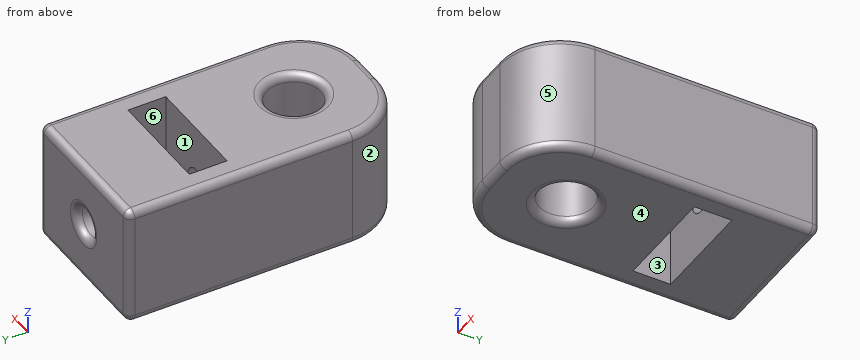
from build123d import *

# Parameters (mm, degrees)
SKETCH1_W           = 12.7
SKETCH1_H           = 24.13
SKETCH1_R           = 2.286
BOSS_EXTRUDE1_DEPTH = 10.16
SKETCH2_R           = 1.27
CUT_EXTRUDE1_DEPTH  = 15.24
FILLET2_R           = 5.08
FILLET1_R           = 0.635
SKETCH3_W           = 8.89
SKETCH3_H           = 3.19532
CUT_EXTRUDE2_DEPTH  = 30.099355663


with BuildPart() as part:
    # Sketch1 → Boss-Extrude1 (new body)
    with BuildSketch(Plane.XY):
        with Locations((6.35, 12.065)):
            Rectangle(SKETCH1_W, SKETCH1_H)
        with Locations((6.35, 6.35)):
            Circle(SKETCH1_R, mode=Mode.SUBTRACT)
    extrude(amount=BOSS_EXTRUDE1_DEPTH)

    # Sketch2 → Cut-Extrude1 (cut)
    with BuildSketch(Plane(origin=(0, 24.13, 0), x_dir=(1, 0, 0), z_dir=(0, 1, 0))):
        with Locations(Location((6.35, -5.08, 0), (0, 0, 270))):
            Circle(SKETCH2_R)
    extrude(amount=-CUT_EXTRUDE1_DEPTH, mode=Mode.SUBTRACT)

    # Fillet2
    fillet2_edges = [part.edges().sort_by_distance(p)[0] for p in [
        (12.7, 0, 5.08),
        (0, 0, 5.08),
    ]]
    fillet(fillet2_edges, radius=FILLET2_R)

    # Fillet1
    fillet1_edges = [part.edges().sort_by_distance(p)[0] for p in [
        (4.064, 6.35, 0),
        (4.064, 6.35, 10.16),
        (6.35, 24.13, 10.16),
        (6.35, 24.13, 3.81),
        (12.7, 14.605, 0),
        (12.7, 14.605, 10.16),
        (6.35, 0, 0),
        (1.487897552, 1.487897552, 0),
        (11.212102448, 1.487897552, 0),
        (6.35, 0, 10.16),
        (1.487897552, 1.487897552, 10.16),
        (11.212102448, 1.487897552, 10.16),
        (0, 14.605, 10.16),
        (6.35, 24.13, 0),
        (0, 14.605, 0),
        (0, 24.13, 5.08),
        (12.7, 24.13, 5.08),
    ]]
    fillet(fillet1_edges, radius=FILLET1_R)

    # Sketch3 → Cut-Extrude2 (cut, through all)
    with BuildSketch(Plane(origin=(0, 0, 0), x_dir=(-1, 0, 0), z_dir=(0, 0, -1))):
        with Locations((-6.35, 16.18234)):
            Rectangle(SKETCH3_W, SKETCH3_H)
    extrude(amount=-CUT_EXTRUDE2_DEPTH, mode=Mode.SUBTRACT)


solid = part.part
Geometry check sheet. Reference: the model listing, model coordinates, mm. Face numbers are marked on the shaded views. A direction names the side the tool comes from. Round coordinates to 2 decimals unless told otherwise and drop trailing zeros. Loops run counter-clockwise (first coordinate to the right, second up) from the corner with the lowest first, then second, coordinate; pieces in that order, holes last. Notation, with made-up numbers: (66.5, 39.25) - (114.5, 39.25) arc R19 ccw to (114.5, 67.25) - close; hole circle Ø4 at (-30, -35). An arc over 180 degrees is marked (long way). One line per question, with ' | ' between items. Start each with the question number.
1. Depth check by flat-ended pin: pin 1 (3.5 mm diameter, centred on x = 6.35, z = 5.08, fed in from +Y); pin 2 (1 mm diameter, centred on x = 10, z = 3, fed in from -Y). Enter the tip coordinate at first touch or a pass-through.
2. Draft check along X on the marked faces 1, 2, 3 and 4. Enter one of: released by +X, released by -X, zero draft, split by the parting line, or undercut.
3. Cross-section at B-B on z = 5.08. Record the cut outline in (x, y) (3 decimals), then the cut area to 3 significant figures.
4. Cross-section at D-D on y = 21.75. Record the cut outline in (x, z) (3 decimals).
5. Cross-section at C-C on x = 6.35. State how many separate pieces and enclosed holes the cut face has, then the cut area to 3 significant figures.
6. Cross-section at A-A on y = 6.35. Record the cut outline in (x, z) (3 decimals).
7. Scan lines: line 1 (Y direction, x = 4.75, z = 1.5); line 2 (Y direction, x = 6.5, z = 6.5); line 3 (X direction, y = 15, z = 3.75) (3 decimals). Record each from-to range of solid material in increasing order. Write a range as [from, to].
8. Tool access check on the marked faces 5 and 6. Record the directions out of +Z, -Z, +X, -X, +Y, -Y that give a thin tool (end or side, any length) a straight path to the whole face; none if there is none.
Taken from the geometry:
1) pin 1: y = 24.11 | pin 2: y = 0.36
2) face 1: undercut | face 2: released by -X | face 3: undercut | face 4: zero draft
3) outline: (0, 5.08) arc R5.08 ccw to (5.08, 0) - (7.62, 0) arc R5.08 ccw to (12.7, 5.08) - (12.7, 23.495) arc R0.635 ccw to (12.065, 24.13) - (8.255, 24.13) arc R0.635 ccw to (7.62, 23.495) - (7.62, 17.78) - (10.795, 17.78) - (10.795, 14.585) - (7.62, 14.585) - (7.62, 8.89) - (5.08, 8.89) - (5.08, 14.585) - (1.905, 14.585) - (1.905, 17.78) - (5.08, 17.78) - (5.08, 23.495) arc R0.635 ccw to (4.445, 24.13) - (0.635, 24.13) arc R0.635 ccw to (0, 23.495) - close; hole circle Ø4.572 at (6.35, 6.35) | area: 220 mm²
4) outline: (0, 0.635) arc R0.635 ccw to (0.635, 0) - (12.065, 0) arc R0.635 ccw to (12.7, 0.635) - (12.7, 9.525) arc R0.635 ccw to (12.065, 10.16) - (0.635, 10.16) arc R0.635 ccw to (0, 9.525) - close; hole circle Ø2.54 at (6.35, 5.08)
5) separate pieces: 4 | enclosed holes: 0 | area: 135 mm²
6) outline: (0, 0.635) arc R0.635 ccw to (0.635, 0) - (3.429, 0) arc R0.635 ccw to (4.064, 0.635) - (4.064, 9.525) arc R0.635 ccw to (3.429, 10.16) - (0.635, 10.16) arc R0.635 ccw to (0, 9.525) - close; (8.636, 0.635) arc R0.635 ccw to (9.271, 0) - (12.065, 0) arc R0.635 ccw to (12.7, 0.635) - (12.7, 9.525) arc R0.635 ccw to (12.065, 10.16) - (9.271, 10.16) arc R0.635 ccw to (8.636, 9.525) - close
7) line 1: [0.01, 4.72], [7.98, 14.58], [17.78, 24.13] | line 2: [0, 4.07], [8.63, 14.58], [17.78, 23.91] | line 3: [0, 1.905], [10.795, 12.7]
8) face 5: +Z, -Z, +X, -Y | face 6: +Z, -Z
